Could you check a few things on this model? Use its own coordinates, in mm. A direction names the side the tool comes from. Give positions to 0.01 mm unless a question says otherwise; leave off trailing zeros. Order: outer loops, then holes, each group sorted by start corner. A loop starts at its lowest first (then second) coordinate and runs counter-clockwise, first axis right, second up. Notation, with made-up numbers: (20, -35.5) -> (51, -35.5) arc R10 cw to (51, -22.5) -> close; hole circle Ø5 at (9, 74.25). An arc over 180 degrees is marked (long way). Use one line per item in the form item = value. Start each with the question number.
from build123d import *

# Parameters (mm, degrees)
SKETCH1_W           = 34
SKETCH1_H           = 34
BOSS_EXTRUDE1_DEPTH = 7
CUT_EXTRUDE1_DEPTH  = 4
SKETCH3_R           = 1.5
CUT_EXTRUDE2_DEPTH  = 10
SKETCH4_R           = 1.5
CUT_EXTRUDE3_DEPTH  = 10
SKETCH5_R           = 1.5
CUT_EXTRUDE4_DEPTH  = 10
SKETCH6_R           = 2.5
CUT_EXTRUDE5_DEPTH  = 1


with BuildPart() as part:
    # Sketch1 → Boss-Extrude1 (new body)
    with BuildSketch(Plane(origin=(0, 0, 0), x_dir=(1, 0, 0), z_dir=(0, 1, 0))):
        Rectangle(SKETCH1_W, SKETCH1_H)
    extrude(amount=BOSS_EXTRUDE1_DEPTH)

    # Sketch2 → Cut-Extrude1 (cut)
    with BuildSketch(Plane(origin=(0, 7, 0), x_dir=(1, 0, 0), z_dir=(0, 1, 0))):
        with BuildLine():
            Line((8, 14), (-8, 14))
            ThreePointArc((-8, 14), (-9.757359313, 9.757359313), (-14, 8))
            Line((-14, 8), (-14, -8))
            ThreePointArc((-14, -8), (-9.757359313, -9.757359313), (-8, -14))
            Line((-8, -14), (8, -14))
            ThreePointArc((8, -14), (9.757359313, -9.757359313), (14, -8))
            Line((14, -8), (14, 8))
            ThreePointArc((14, 8), (9.757359313, 9.757359313), (8, 14))
        make_face()
    extrude(amount=-CUT_EXTRUDE1_DEPTH, mode=Mode.SUBTRACT)

    # Sketch3 → Cut-Extrude2 (cut)
    with BuildSketch(Plane.XY.offset(17)):
        with Locations((0, 7)):
            Circle(SKETCH3_R)
    extrude(amount=-CUT_EXTRUDE2_DEPTH, mode=Mode.SUBTRACT)

    # Sketch4 → Cut-Extrude3 (cut)
    with BuildSketch(Plane(origin=(0, 7, 0), x_dir=(1, 0, 0), z_dir=(0, 1, 0))):
        with Locations(Location((-14, 14, 0), (0, 0, 270))):
            Circle(SKETCH4_R)
        with Locations(Location((14, 14, 0), (0, 0, 270))):
            Circle(SKETCH4_R)
        with Locations(Location((14, -14, 0), (0, 0, 270))):
            Circle(SKETCH4_R)
        with Locations(Location((-14, -14, 0), (0, 0, 270))):
            Circle(SKETCH4_R)
    extrude(amount=-CUT_EXTRUDE3_DEPTH, mode=Mode.SUBTRACT)

    # Sketch5 → Cut-Extrude4 (cut)
    with BuildSketch(Plane(origin=(0, 3, 0), x_dir=(1, 0, 0), z_dir=(0, 1, 0))):
        with Locations(Location((0, 0, 0), (0, 0, 270))):
            Circle(SKETCH5_R)
    extrude(amount=-CUT_EXTRUDE4_DEPTH, mode=Mode.SUBTRACT)

    # Sketch6 → Cut-Extrude5 (cut)
    with BuildSketch(Plane(origin=(0, 3, 0), x_dir=(1, 0, 0), z_dir=(0, 1, 0))):
        with Locations(Location((0, 0, 0), (0, 0, 270))):
            Circle(SKETCH6_R)
    extrude(amount=-CUT_EXTRUDE5_DEPTH, mode=Mode.SUBTRACT)


solid = part.part
(1) Imagine slicing it at A-A (x = 0). Write out the boundary of the cut face in (y, z).
(2) We'd pull the mould along X, two halves only. Please class faces 1 (the flat face through (-17, 3, 0)), 2 (the flat face through (17, 3, 0)), 3 (the flat face through (0, 3, -3)), 4 (the flat face through (0, 3, 17)): pulls with the +X half, pulls with the -X half, needs draft (parallel to the pull), parting line crosses it, or undercut.
(3) Imagine slicing it at C-C (y = 1.5). Write out the boundary of the cut face in (x, z), plus the area to 3 significant figures.
(4) I'm going to push flat-ended pins straight in: pin 1 Ø12 at (x, z) = (6.5, -2.5) entering from -Y; pin 2 Ø5 at (x, z) = (-3, -10) entering from +Y; pin 3 Ø4.5 at (x, z) = (0, 0) entering from +Y. Where does each tip first touch, or does it pass through?
(5) Which directions (+Z, -Z, +X, -X, +Y, -Y) give clear straight access to the entire face, cutting with the end or side of a thin tool? Please do faces 5 (the cylindrical face through (0, 5.5, 15.5)), 6 (the cylindrical face through (-13.93, 3.55, -15.5)), 7 (the flat face through (0, 5, -14)).
(6) Please list where these lines run through material, in increasing order: probe 1 along X at (y, z) = (2.75, -14); probe 2 along X at (y, z) = (6, 6).
(7) Imagine slicing it at D-D (z = 7). Write out the boundary of the cut face in (x, y).
(8) Imagine slicing it at B-B (z = 0). Write out the boundary of the cut face in (x, y), plus the area to 3 significant figures.
Calculated:
q1.outline = (0, -17) -> (7, -17) -> (7, -14) -> (3, -14) -> (3, -2.5) -> (2, -2.5) -> (2, -1.5) -> (0, -1.5) -> close; (0, 1.5) -> (2, 1.5) -> (2, 2.5) -> (3, 2.5) -> (3, 14) -> (5.5, 14) -> (5.5, 17) -> (0, 17) -> close
q2.face_1 = pulls with the -X half
q2.face_2 = pulls with the +X half
q2.face_3 = undercut
q2.face_4 = needs draft
q3.outline = (-17, -17) -> (17, -17) -> (17, 17) -> (-17, 17) -> close; hole circle Ø3 at (-14, -14); hole circle Ø3 at (-14, 14); hole circle Ø3 at (0, 0); hole circle Ø3 at (14, -14); hole circle Ø3 at (14, 14)
q3.area = 1,120 mm2
q4.pin_1 = 0
q4.pin_2 = 3
q4.pin_3 = 2
q5.face_5 = +Z, +Y
q5.face_6 = +Y, -Y
q5.face_7 = +Y
q6.probe_1 = -17 to -15.5, -12.5 to 12.5, 15.5 to 17
q6.probe_2 = -17 to -14, 14 to 17
q7.outline = (-17, 0) -> (17, 0) -> (17, 7) -> (14, 7) -> (14, 3) -> (-14, 3) -> (-14, 7) -> (-17, 7) -> close
q8.outline = (-17, 0) -> (-1.5, 0) -> (-1.5, 2) -> (-2.5, 2) -> (-2.5, 3) -> (-14, 3) -> (-14, 7) -> (-17, 7) -> close; (1.5, 0) -> (17, 0) -> (17, 7) -> (14, 7) -> (14, 3) -> (2.5, 3) -> (2.5, 2) -> (1.5, 2) -> close
q8.area = 115 mm2
